Could you check a few things on this model? Use its own coordinates, in mm. Face numbers are marked on the shaded views. A direction names the side the tool comes from. Give positions to 0.01 mm unless a question says otherwise; leave off trailing zeros. Order: outer loops, then holes, each group sorted by start corner. A loop starts at its lowest first (then second) coordinate and runs counter-clockwise, first axis right, second up.
(1) On a 3-axis mill with a long thin cutter (end or side, diameter ignored), from which of +Z, -Z, +X, -X, +Y, -Y can I reach the whole of each face in a straight line? I mean the marked faces 1 and 2. Say none if no direction works.
(2) Imagine slicing it at B-B, the plane x = -8.5. Write out the boundary of the cut face in (y, z).
(3) If we mould it in two halves opening along Y, with no side actions, what happens to the marked faces 3, 4, 5 and 6? For each: released by +Y, released by -Y, zero draft, split by the parting line, or undercut.
(4) Imagine slicing it at C-C, the plane y = 32.5. Write out the boundary of the cut face in (x, z), then the cut area to 3 significant figures.
(5) Will these pins go through, and if not, where does the flat tip stop? pin 1 (1.6 mm diameter, centred on y = -44, z = 6, fed in from +X); pin 2 (1.2 mm diameter, centred on x = 2.5, z = -0.5, fed in from +Y); pin 3 (8 mm diameter, centred on x = 17.5, y = 7.5, fed in from +Z).
(6) Imagine slicing it at A-A, the plane z = 6. Write out the boundary of the cut face in (x, y).
(7) Imagine slicing it at D-D, the plane z = 2.25. Write out the boundary of the cut face in (x, y).
(8) If I drill on probe 1 along Y at (x, z) = (25, 2.25); probe 2 along X at (y, z) = (-25.5, 4.5); probe 3 along Y at (x, z) = (4.5, 0.75), over which ranges is the centre line in solid material (lowest first)?
from build123d import *

# Parameters (mm, degrees)
F0_W     = 55
F0_H     = 86.6
F1_DEPTH = 8
F2_R     = 2
F3_T     = 1.44
F4_W     = 15
F4_H     = 3
F5_DEPTH = 48.1
F6_W     = 15
F6_H     = 1.44
F7_DEPTH = 25


with BuildPart() as f1:
    # F0 (on Top) → F1 (new body)
    with BuildSketch(Plane.XY):
        Rectangle(F0_W, F0_H)
    extrude(amount=F1_DEPTH)

    # F2
    f2_edges = [f1.edges().sort_by_distance(p)[0] for p in [
        (-27.5, -43.3, 4),
        (27.5, -43.3, 4),
        (27.5, 43.3, 4),
        (-27.5, 43.3, 4),
    ]]
    fillet(f2_edges, radius=F2_R)

    # F3
    f3_openings = [f1.faces().sort_by_distance(p)[0] for p in [
        (0, 0, 8),
    ]]
    offset(amount=F3_T, openings=f3_openings, kind=Kind.INTERSECTION)

    # F4 (on Front) → F5 (cut, symmetric)
    with BuildSketch(Plane.XZ):
        with Locations((0, 6.5)):
            Rectangle(F4_W, F4_H)
    extrude(amount=F5_DEPTH, both=True, mode=Mode.SUBTRACT)

    # F6 (on face) → F7 (cut)
    with BuildSketch(Plane(origin=(0, 0, -1.44), x_dir=(1, 0, 0), z_dir=(0, 0, -1))):
        with Locations((0, -44.02)):
            Rectangle(F6_W, F6_H)
    extrude(amount=-F7_DEPTH, mode=Mode.SUBTRACT)


solid = f1.part
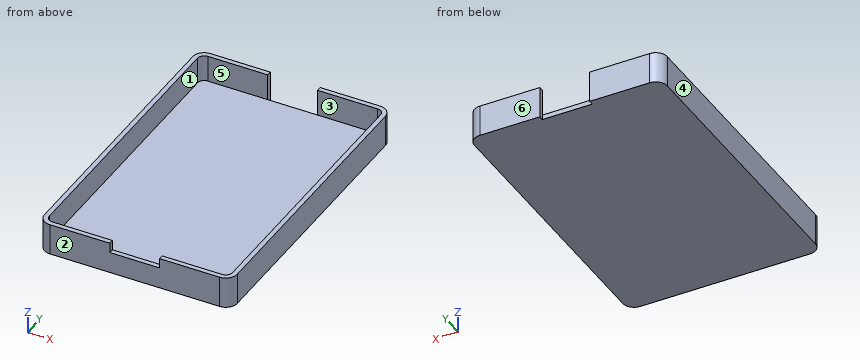
Answer block:
1. face 1: +Z
1. face 2: +Z, -Z, +X, -X, -Y
2. outline: (-44.74, -1.44) - (44.74, -1.44) - (44.74, 8) - (43.3, 8) - (43.3, 0) - (-43.3, 0) - (-43.3, 8) - (-44.74, 8) - close
3. face 3: undercut
3. face 4: zero draft
3. face 5: undercut
3. face 6: released by +Y
4. outline: (-28.94, -1.44) - (28.94, -1.44) - (28.94, 8) - (27.5, 8) - (27.5, 0) - (-27.5, 0) - (-27.5, 8) - (-28.94, 8) - close
4. area: 106 mm2
5. pin 1: stops at x = 28.37
5. pin 2: stops at y = 43.3
5. pin 3: stops at z = 0
6. outline: (-28.94, -41.3) arc R3.44 ccw to (-25.5, -44.74) - (-7.5, -44.74) - (-7.5, -43.3) - (-25.5, -43.3) arc R2 cw to (-27.5, -41.3) - (-27.5, 41.3) arc R2 cw to (-25.5, 43.3) - (-7.5, 43.3) - (-7.5, 44.74) - (-25.5, 44.74) arc R3.44 ccw to (-28.94, 41.3) - close; (7.5, -44.74) - (25.5, -44.74) arc R3.44 ccw to (28.94, -41.3) - (28.94, 41.3) arc R3.44 ccw to (25.5, 44.74) - (7.5, 44.74) - (7.5, 43.3) - (25.5, 43.3) arc R2 cw to (27.5, 41.3) - (27.5, -41.3) arc R2 cw to (25.5, -43.3) - (7.5, -43.3) - close
7. outline: (-28.94, -41.3) arc R3.44 ccw to (-25.5, -44.74) - (25.5, -44.74) arc R3.44 ccw to (28.94, -41.3) - (28.94, 41.3) arc R3.44 ccw to (25.5, 44.74) - (7.5, 44.74) - (7.5, 43.3) - (25.5, 43.3) arc R2 cw to (27.5, 41.3) - (27.5, -41.3) arc R2 cw to (25.5, -43.3) - (-25.5, -43.3) arc R2 cw to (-27.5, -41.3) - (-27.5, 41.3) arc R2 cw to (-25.5, 43.3) - (-7.5, 43.3) - (-7.5, 44.74) - (-25.5, 44.74) arc R3.44 ccw to (-28.94, 41.3) - close
8. probe 1: y = -44.74 to -43.3, 43.3 to 44.74
8. probe 2: x = -28.94 to -27.5, 27.5 to 28.94
8. probe 3: y = -44.74 to -43.3
